Verification items for this drawing (mm, ordinates from the low corner). A direction names the side the tool comes from. Coordinates: 2 decimals unless noted, no trailing zeros. Write each loop counter-clockwise with the first axis right and the second up, starting at its lowest first coordinate (ties: lowest second). Pieces come first, ordered by that corner, then holes. Notation, with made-up numbers: M 69.25,18.5 L 110.25,18.5 A21 cw 110.25,39.5 Z; hole C 31.5,-20 d3. An arc over 180 degrees is marked long. Answer as CSV lines item,"result". Start each with the question number.
1) Material ranges on L1, parallel to Z at x = 25.15, y = 24.15; L2, parallel to Z at x = 25.15, y = 12.5; L3, parallel to Z at x = 25.15, y = 18.3, recorded low to high. Write a range as [from, to].
2) Section check B-B (z = 25.15). Record the cut outline in (x, y).
3) Section check D-D (y = 4). Record the cut outline in (x, z), and give its area (3 significant figures).
4) Section check A-A (x = 25.15). Record the cut outline in (y, z).
5) Access from +Z, -Z, +X, -X, +Y, -Y to the whole of each face (thin tool, end or side, straight path). Record for the marked faces 1 and 2.
6) Section check C-C (y = 19). Record the cut outline in (x, z), and give its area (3 significant figures).
7) Go/stop test with flat-tipped pins: pin 1 Ø5 at (x, z) = (22.5, 23) entering from +Y; pin 2 Ø6 at (y, z) = (3.5, 15.5) entering from +X; pin 3 Ø1.5 at (y, z) = (19, 23.5) entering from +X. Record where each tip stops, or that it passes through.
8) Draft check along Z on the marked faces 3, 4 and 5. Enter one of: +Z half, -Z half, draft (parallel to the pull), parting line (faces both ways), or undercut.
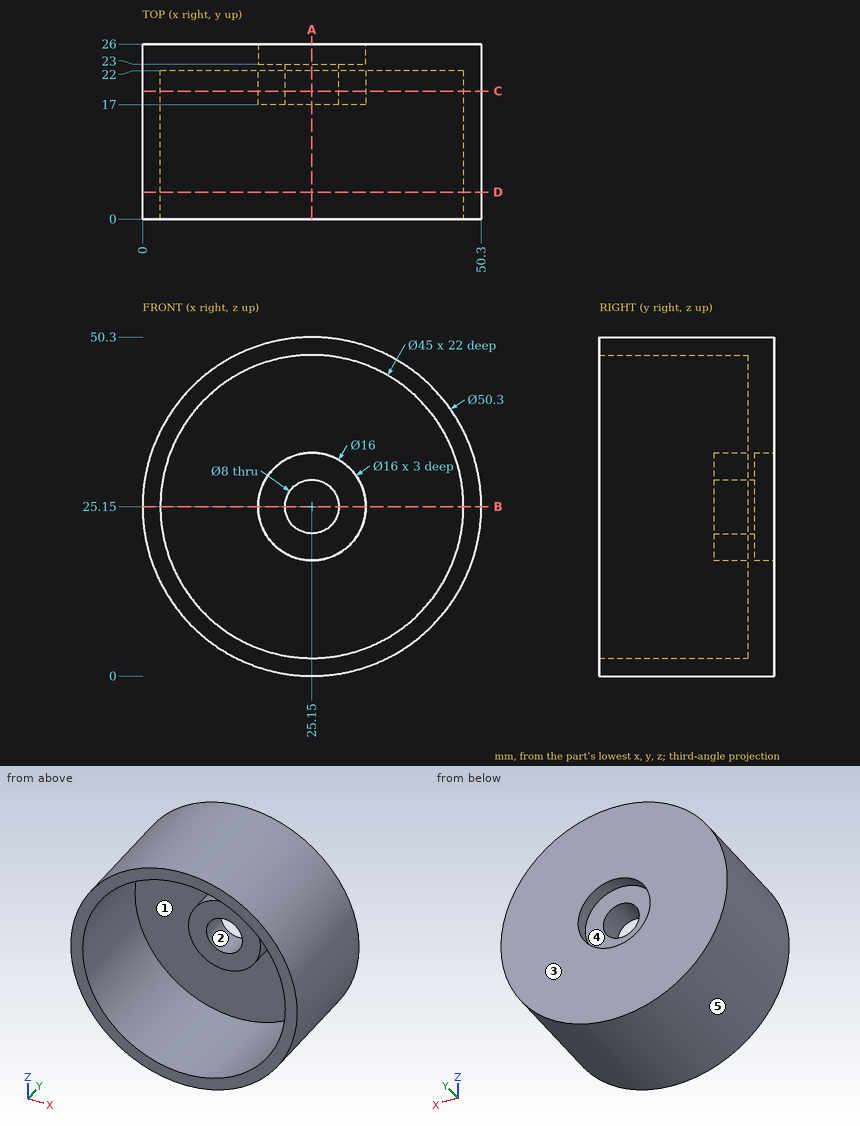
Results found:
1,L1,"z = [0, 17.15], [33.15, 50.3]"
1,L2,"z = [0, 2.65], [47.65, 50.3]"
1,L3,"z = [0, 2.65], [17.15, 21.15], [29.15, 33.15], [47.65, 50.3]"
2,outline,"M 0,0 L 2.65,0 L 2.65,22 L 17.15,22 L 17.15,17 L 21.15,17 L 21.15,23 L 17.15,23 L 17.15,26 L 0,26 Z; M 29.15,17 L 33.15,17 L 33.15,22 L 47.65,22 L 47.65,0 L 50.3,0 L 50.3,26 L 33.15,26 L 33.15,23 L 29.15,23 Z"
3,outline,"C 25.15,25.15 d50.3; hole C 25.15,25.15 d45"
3,area,"397 mm2"
4,outline,"M 0,0 L 26,0 L 26,17.15 L 23,17.15 L 23,21.15 L 17,21.15 L 17,17.15 L 22,17.15 L 22,2.65 L 0,2.65 Z; M 0,47.65 L 22,47.65 L 22,33.15 L 17,33.15 L 17,29.15 L 23,29.15 L 23,33.15 L 26,33.15 L 26,50.3 L 0,50.3 Z"
5,face 1,"-Y"
5,face 2,"+Y, -Y"
6,outline,"C 25.15,25.15 d50.3; C 25.15,25.15 d16; hole C 25.15,25.15 d45; hole C 25.15,25.15 d8"
6,area,"547 mm2"
7,pin 1,"stops at y = 23"
7,pin 2,"stops at x = 49.4"
7,pin 3,"stops at x = 50.28"
8,face 3,"draft"
8,face 4,"undercut"
8,face 5,"parting line"
